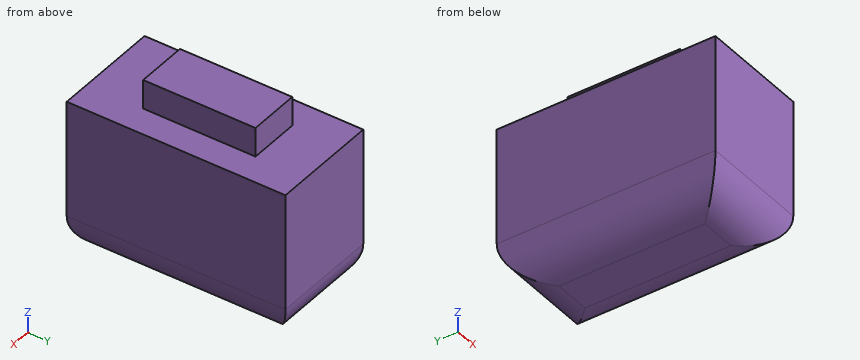
from build123d import *

# Parameters (mm, degrees)
SKETCH_3_W           = 3
SKETCH_3_H           = 6
EXTRUDE_2_DEPTH      = 3.5
SKETCH_4_OUTSIDE_W   = 6.514
SKETCH_4_OUTSIDE_H   = 9.514
SKETCH_4_OUTSIDE_W_2 = 1.417406922
SKETCH_4_OUTSIDE_H_2 = 3.080497711
CUT_EXTRUDE_1_DEPTH  = 0.8
SKETCH_9_W           = 3
SKETCH_9_H           = 6
EXTRUDE_5_DEPTH      = 1.5
FILLET_2_R           = 1


with BuildPart() as part:
    # 草图3 → 凸台-拉伸2 (new body)
    with BuildSketch(Plane.XY):
        with Locations((-0.538539978, -1.817017803)):
            Rectangle(SKETCH_3_W, SKETCH_3_H)
    extrude(amount=EXTRUDE_2_DEPTH)

    # 草图4 outside → 切除-拉伸1 (cut)
    with BuildSketch(Plane.XY.offset(3.5)):
        with Locations((-0.539, -1.817)):
            Rectangle(SKETCH_4_OUTSIDE_W, SKETCH_4_OUTSIDE_H)
        with Locations((-0.530790021, -1.736698078)):
            Rectangle(SKETCH_4_OUTSIDE_W_2, SKETCH_4_OUTSIDE_H_2, mode=Mode.SUBTRACT)
    extrude(amount=-CUT_EXTRUDE_1_DEPTH, mode=Mode.SUBTRACT)

    # 草图9 → 凸台-拉伸5 (add)
    with BuildSketch(Plane(origin=(0, 0, 0), x_dir=(-1, 0, 0), z_dir=(0, 0, -1))):
        with Locations((0.538539978, -1.817017803)):
            Rectangle(SKETCH_9_W, SKETCH_9_H)
    extrude(amount=EXTRUDE_5_DEPTH)

    # 圆角2
    fillet_2_edges = [part.edges().sort_by_distance(p)[0] for p in [
        (0.961460022, -1.817017803, -1.5),
        (-0.538539978, -4.817017803, -1.5),
        (-2.038539978, -1.817017803, -1.5),
        (-0.538539978, 1.182982197, -1.5),
    ]]
    fillet(fillet_2_edges, radius=FILLET_2_R)


solid = part.part
Design review of the part built by this model. Coordinates are the model's own, in mm. Round coordinates to 2 decimals unless told otherwise and drop trailing zeros. Loops run counter-clockwise (first coordinate to the right, second up) from the corner with the lowest first, then second, coordinate; pieces in that order, holes last. Notation, with made-up numbers: (-29, -39.75) - (-22, -39.75) arc R16 ccw to (-22, -19.75) - close; hole circle Ø6 at (-5.5, 37.25). An arc over 180 degrees is marked (long way). One line per item, written item: value. Start each with the question number.
1) Consider section C-C on x = 0.35. Give the boundary of the cut face in (y, z).
2) Consider section A-A on y = -1.95. Give the boundary of the cut face in (x, z).
3) Consider section D-D on y = -3.75. Give the boundary of the cut face in (x, z).
4) To check wall thickness, follow L1, parallel to Z at x = -1.05, y = 0.25; L2, parallel to Y at x = -0.95, z = 3; L3, parallel to X at y = -0.8, z = -0.9. State the ranges of each line that lie inside material, in increasing order. Write a range as from..to.
5) Consider section B-B on z = 2.9. Give the boundary of the cut face in (x, y).
Reported:
1. outline: (-4.82, -0.5) arc R1 ccw to (-4.21, -1.42) - (0.57, -1.42) arc R1 ccw to (1.18, -0.5) - (1.18, 2.7) - (-4.82, 2.7) - close
2. outline: (-2.04, -0.5) arc R1 ccw to (-1.04, -1.5) - (-0.04, -1.5) arc R1 ccw to (0.96, -0.5) - (0.96, 2.7) - (0.18, 2.7) - (0.18, 3.5) - (-1.24, 3.5) - (-1.24, 2.7) - (-2.04, 2.7) - close
3. outline: (-2.04, -0.5) arc R1 ccw to (-1.04, -1.5) - (-0.04, -1.5) arc R1 ccw to (0.96, -0.5) - (0.96, 2.7) - (-2.04, 2.7) - close
4. L1: z = -1.5..2.7
4. L2: y = -3.28..-0.2
4. L3: x = -1.96..0.88
5. outline: (-1.24, -3.28) - (0.18, -3.28) - (0.18, -0.2) - (-1.24, -0.2) - close
